Geometry: see drawing. Coordinates: mm, zero at the bounding-box minimum. A direction names the side the tool comes from. Coordinates: 2 decimals unless noted, no trailing zeros. Write each loop counter-clockwise with the first axis right and the second up, starting at its lowest first coordinate (ties: lowest second). Pieces come first, ordered by that corner, then holes. Notation, with made-up numbers: (-15, 61) - (8, 61) arc R8 ccw to (8, 67) - close; hole circle Ø4 at (54.25, 54.5). An arc over 180 degrees is marked (long way). Use a Markdown table: item, result. Add a question column.
Q1. Section query C-C (z = 25). Return the cut outline in (x, y), then the cut area to 3 significant figures.
Q2. Material intervals for probe 1 along X at (y, z) = (137, 37); probe 2 along Z at (x, y) = (124, 25); probe 3 along Y at (x, z) = (29.5, 41), sorted ascending. Write a range as from..to.
Q3. Pin query (flat end, axial travel): P1, Ø12, axis at x = 21, z = 38, coming from the -Y side; P2, Ø10.5, axis at y = 25, z = 25, coming from the +X side. Return the tip coordinate at first contact, or that it passes through.
Q4. Mould query, pull axis X, two halves, no side actions, for the marked faces 3, 4, 5 and 6. Classes: released by +X, released by -X, zero draft, split by the parting line, or undercut.
Q5. Section query A-A (x = 65). Return the cut outline in (y, z).
Q6. Set-up query: the marked faces 1 and 2. Return all of +Z, -Z, +X, -X, +Y, -Y with unobstructed straight access to the full face (end or side cutting, diameter ignored); none if empty.
Q7. Section query D-D (y = 25). Return the cut outline in (x, z), then the cut area to 3 significant figures.
Q8. Section query B-B (y = 178.5). Return the cut outline in (x, z), then the cut area to 3 significant figures.
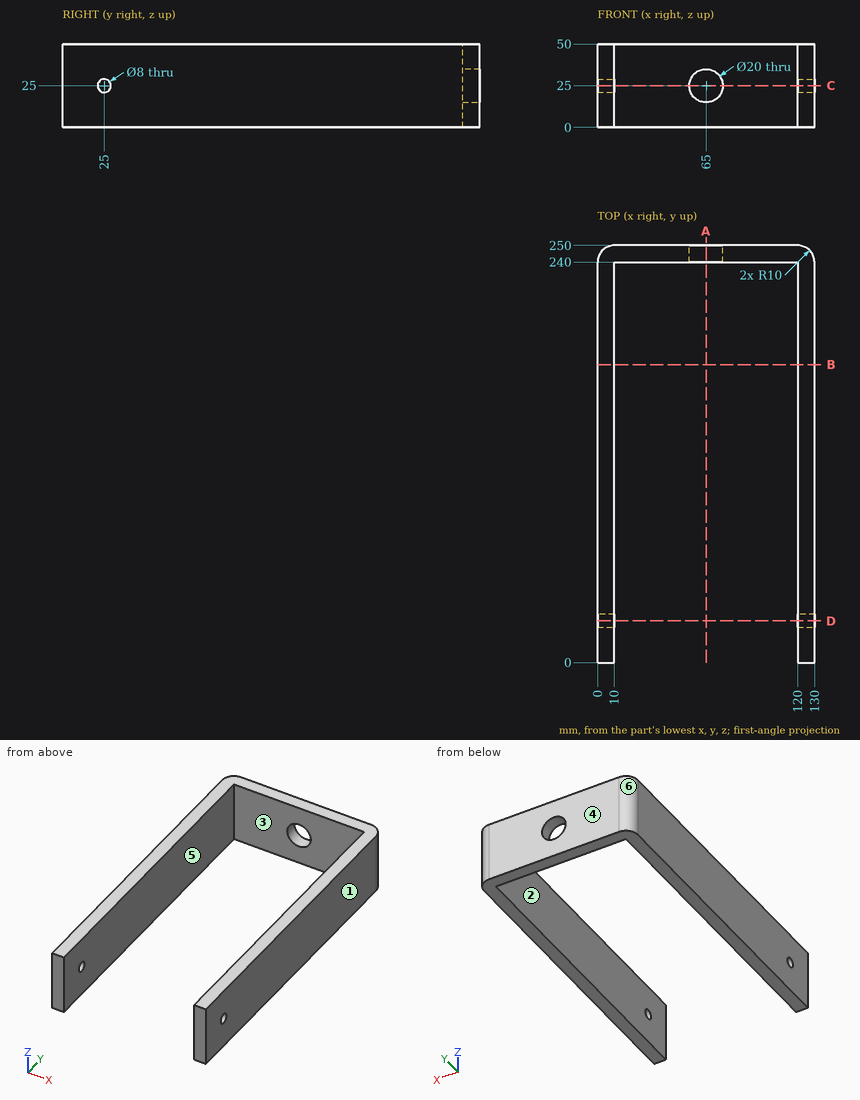
Values follow:
| question | item | result |
|---|---|---|
| 1 | outline | (0, 0) - (10, 0) - (10, 21) - (0, 21) - close; (0, 29) - (10, 29) - (10, 240) - (55, 240) - (55, 250) - (10, 250) arc R10 ccw to (0, 240) - close; (75, 240) - (120, 240) - (120, 29) - (130, 29) - (130, 240) arc R10 ccw to (120, 250) - (75, 250) - close; (120, 0) - (130, 0) - (130, 21) - (120, 21) - close |
| 1 | area | 5,700 mm2 |
| 2 | probe 1 | 0..10, 120..130 |
| 2 | probe 2 | 0..21, 29..50 |
| 2 | probe 3 | 240..250 |
| 3 | P1 | y = 240 |
| 3 | P2 | x = 130 |
| 4 | face 3 | undercut |
| 4 | face 4 | zero draft |
| 4 | face 5 | undercut |
| 4 | face 6 | released by -X |
| 5 | outline | (240, 0) - (250, 0) - (250, 15) - (240, 15) - close; (240, 35) - (250, 35) - (250, 50) - (240, 50) - close |
| 6 | face 1 | +Z, -Z, +X, +Y, -Y |
| 6 | face 2 | +Z, -Z, -Y |
| 7 | outline | (0, 0) - (10, 0) - (10, 21) - (0, 21) - close; (0, 29) - (10, 29) - (10, 50) - (0, 50) - close; (120, 0) - (130, 0) - (130, 21) - (120, 21) - close; (120, 29) - (130, 29) - (130, 50) - (120, 50) - close |
| 7 | area | 840 mm2 |
| 8 | outline | (0, 0) - (10, 0) - (10, 50) - (0, 50) - close; (120, 0) - (130, 0) - (130, 50) - (120, 50) - close |
| 8 | area | 1,000 mm2 |
